CAD build for the part. Positions are in the model's coordinates, mm. Face numbers are marked on the shaded views. Give positions to 0.01 mm unless a question says otherwise; leave off trailing zeros. Write each loop counter-clockwise with the first axis right and the second up, starting at its lowest first coordinate (ties: lowest second). Pieces come first, ordered by that corner, then holes. Notation, with made-up numbers: (88.5, 0) -> (111.5, 0) arc R24 cw to (111.5, 25) -> close; hole circle Ø5 at (-3.5, 38). An arc over 180 degrees is marked (long way). Use one line per item in the form item = value. Start each with the question number.
from build123d import *

# Parameters (mm, degrees)
SKETCH005_R      = 1.3
EXTRUDE003_DEPTH = 20
EXTRUDE039_DEPTH = 4
EXTRUDE042_DEPTH = 0.8
EXTRUDE002_DEPTH = 6
EXTRUDE037_DEPTH = 2


with BuildPart() as sweep001:
    # Sweep001: sweep along a path in Sketch034
    with BuildLine(Plane.XZ.offset(10)) as sweep001_path:
        Line((32, 12), (32, 48.4))
        ThreePointArc((32, 48.4), (30.652691, 51.652691), (27.4, 53))
        Line((27.4, 53), (-20, 53))
    # Sketch035 → Sweep001 (sweep)
    with BuildSketch(Plane.YZ):
        Polygon((5.3, 51.4), (3.7, 53), (3.7, 54), (6, 54), (6, 51.4), align=None)
    sweep(path=sweep001_path.line)


with BuildPart() as fusion030:
    # Sketch005 → Extrude003 (new body)
    with BuildSketch(Plane.XZ.offset(5)):
        with Locations((27.4, 48.5)):
            Circle(SKETCH005_R)
    extrude(amount=-EXTRUDE003_DEPTH)


with BuildPart() as fusion030_1:
    # Extrude003 placement: moved
    add(fusion030.part.moved(Location((0, -4, 0))))

    # Fusion030: union Sweep001
    add(sweep001.part)


with BuildPart() as top003:
    # Sketch028 → Extrude039 (new body)
    with BuildSketch(Plane.XZ.offset(10)):
        with BuildLine():
            ThreePointArc((32, 48.4), (30.652691, 51.652691), (27.4, 53))
            Line((27.4, 53), (-20, 53))
            Line((-20, 53), (-20, 51))
            Line((-20, 51), (27.4, 51))
            ThreePointArc((30, 48.4), (29.238478, 50.238478), (27.4, 51))
            Line((30, 23), (30, 48.4))
            Line((32, 23), (30, 23))
            Line((32, 48.4), (32, 23))
        make_face()
    extrude(amount=EXTRUDE039_DEPTH)


with BuildPart() as top003_1:
    # Extrude039 placement: moved
    add(top003.part.moved(Location((0, 14.5, 0))))


with BuildPart() as top002:
    # Sketch031 → Extrude042 (new body)
    with BuildSketch(Plane.XZ.offset(10)):
        with BuildLine():
            ThreePointArc((32, 48.4), (30.652691, 51.652691), (27.4, 53))
            Line((27.4, 53), (-20, 53))
            Line((-20, 53), (-20, 23))
            Line((-20, 23), (32, 23))
            Line((32, 48.4), (32, 23))
        make_face()
    extrude(amount=EXTRUDE042_DEPTH)


with BuildPart() as top002_1:
    # Extrude042 placement: moved
    add(top002.part.moved(Location((0, 15.3, 0))))


with BuildPart() as screw_hole_top:
    # Sketch004 → Extrude002 (new body)
    with BuildSketch(Plane.XZ.offset(10)):
        with BuildLine():
            ThreePointArc((23.975091, 51), (24.359441, 45.359441), (30, 44.975091))
            Line((30, 44.975091), (30, 48.4))
            ThreePointArc((30, 48.4), (29.238478, 50.238478), (27.4, 51))
            Line((23.975091, 51), (27.4, 51))
        make_face()
    extrude(amount=-EXTRUDE002_DEPTH)


with BuildPart() as screw_hole_top_1:
    # Extrude002 placement: moved
    add(screw_hole_top.part.moved(Location((0, 8.5, 0))))


with BuildPart() as top:
    # Sketch029 → Extrude037 (new body)
    with BuildSketch(Plane.XZ.offset(10)):
        with BuildLine():
            ThreePointArc((30.9, 48.4), (29.874874, 50.874874), (27.4, 51.9))
            Line((27.4, 51.9), (-20, 51.9))
            Line((-20, 51.9), (-20, 51))
            Line((-20, 51), (27.4, 51))
            ThreePointArc((30, 48.4), (29.238478, 50.238478), (27.4, 51))
            Line((30, 23), (30, 48.4))
            Line((30.9, 23), (30, 23))
            Line((30.9, 48.4), (30.9, 23))
        make_face()
    extrude(amount=EXTRUDE037_DEPTH)


with BuildPart() as top_1:
    # Extrude037 placement: moved
    add(top.part.moved(Location((0, 10.5, 0))))

    # Fusion028: union top003, top002, screw hole top
    add(top003_1.part)
    add(top002_1.part)
    add(screw_hole_top_1.part)

    # Cut024: cut Fusion030
    add(fusion030_1.part, mode=Mode.SUBTRACT)


with BuildPart() as part_mirroring001:
    # Part__Mirroring001: instance of top
    add(top_1.part.mirror(Plane(origin=(0, 0, 0), x_dir=(0, 1, 0), z_dir=(0, 0, 1))))


solid = part_mirroring001.part
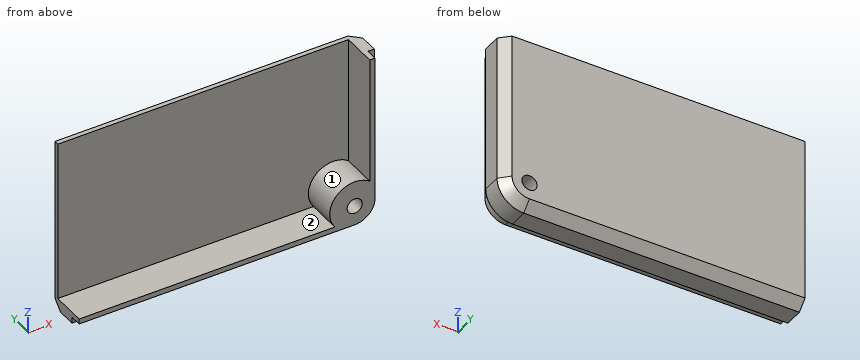
1) Cut at D-D (y = 2.5). Give the cut face in (x, z), and give its area (3 significant figures).
2) Cut at C-C (x = -7). Give the cut face in (y, z).
3) Pin check, flat tips, straight feed: pin 1 (5 mm diameter, centred on x = 17, z = -29.5, fed in from -Y); pin 2 (3 mm diameter, centred on y = 2, z = -30, fed in from -X); pin 3 (1.5 mm diameter, centred on x = 18, y = 2.5, fed in from +Z). Stop position of each tip, or through.
4) Cut at B-B (z = -37.5). Give the cut face in (x, y).
5) Wall check: line 1 along Z through (x, y) = (27.4, 1.5); line 2 along X through (y, z) = (2.25, -48.5); line 3 along X through (y, z) = (0, -48.5). Give the ranges that are in metal, low to high. Write a range as from..to.
6) Cut at A-A (y = 0). Give the cut face in (x, z).
7) Two-plate mould, pull along X, no slides. Class the marked faces 1 and 2: released by +X, released by -X, zero draft, split by the parting line, or undercut.
Final values:
q1.outline = (-20, -53) -> (27.4, -53) arc R4.6 ccw to (32, -48.4) -> (32, -23) -> (30, -23) -> (30, -44.98) arc R4.3 ccw to (23.98, -51) -> (-20, -51) -> close; hole circle Ø2.6 at (27.4, -48.5)
q1.area = 192 mm^2
q2.outline = (-1.5, -51.9) -> (0.5, -51.9) -> (0.5, -53) -> (3.7, -53) -> (5.3, -51.4) -> (5.3, -23) -> (4.5, -23) -> (4.5, -51) -> (-1.5, -51) -> close
q3.pin_1 = 4.5
q3.pin_2 = 30
q3.pin_3 = -51
q4.outline = (-20, 4.5) -> (30, 4.5) -> (30, -1.5) -> (30.9, -1.5) -> (30.9, 0.5) -> (32, 0.5) -> (32, 3.7) -> (30.4, 5.3) -> (-20, 5.3) -> close
q5.line_1 = -53..-49.8, -47.2..-44.1
q5.line_2 = 23.1..26.1, 28.7..32
q5.line_3 = 23.1..26.1, 28.7..30.9
q6.outline = (-20, -51.9) -> (27.4, -51.9) arc R3.5 ccw to (30.9, -48.4) -> (30.9, -23) -> (30, -23) -> (30, -44.98) arc R4.3 ccw to (23.98, -51) -> (-20, -51) -> close; hole circle Ø2.6 at (27.4, -48.5)
q7.face_1 = undercut
q7.face_2 = zero draft
